Autodesk Inventor part; units mm, degrees
ref_plane "Work Plane1" through (0, 0, 23.8252) normal (0, 0, 1) x (1, 0, 0)
sketch "Sketch1" plane through (0, 0, 0) normal (0, 1, 0) x (-1, 0, 0)
  circle A0 centre (0, 0) radius 30.48
  dimension "d0" = 60.96
extrude "Extrusion1" add sketch "Sketch1" along normal blind 25.4
sketch "Sketch2" plane through (0, 25.4, 0) normal (0, 1, 0) x (1, 0, 0)
  circle A0 centre (0, 0) radius 30.48
  circle A1 centre (0, 0) radius 15.24
  dimension "d3" = 30.48
extrude "Extrusion2" cut sketch "Sketch2" against normal blind 20.828
hole "Hole1" at (0, 25.4, 0) direction (0, -1, 0) diameter 22.225 end through all
ref_plane "Work Plane1" through (0, 0, 23.8252) normal (0, 0, 1) x (1, 0, 0)
hole "Hole2" at (0, 0, 23.8252) direction (0, 1, 0) diameter 5.08 end through all
pattern_circular "Circular Pattern1" count 6 over 360 about axis through (0, 25.4, 0) along (0, -1, 0) of "Hole2"
properties part number ".875 Bearing Hub"
Could you check a few things on this model? Use its own coordinates, in mm. Coordinates: 2 decimals unless noted, no trailing zeros. Write each loop counter-clockwise with the first axis right and the second up, starting at its lowest first coordinate (ties: lowest second). Pieces come first, ordered by that corner, then holes. Notation, with made-up numbers: (-29.75, 25) - (-0.75, 25) arc R24 ccw to (-0.75, 41) - close; hole circle Ø11 at (-0.75, -37). An arc over 180 degrees is marked (long way). Put each result on its own line as item: value. Start each with the question number.
Q1. I want a section at B-B on z = 0. Write out the boundary of the cut face in (x, y).
Q2. I'm going to push flat-ended pins straight in: P1, Ø1, axis at x = 0.5, y = 17.5, coming from the +Z side; P2, Ø6.5, axis at x = 20.63, z = -11.91, coming from the +Y side. Where does each tip first touch, or does it pass through?
Q3. I want a section at C-C on y = 15.5. Write out the boundary of the cut face in (x, z) (1 decimal), plus the area to 3 significant figures.
Q4. Please list where these lines run through material, in increasing order: L1, parallel to Z at x = 0, y = 12.5; L2, parallel to Y at x = 28, z = -11; L3, parallel to X at y = 11, z = 6.
Q5. I want a section at D-D on x = -7. Write out the boundary of the cut face in (y, z).
Q6. I want a section at A-A on x = 0. Write out the boundary of the cut face in (y, z).
Q7. Thinking about a two-plate mould opening in Z: for faces 1 (the cylindrical face through (-3.3, 15.13, 14.88)), 2 (the flat face through (-7, 4.572, -14)), 3 (the cylindrical face through (23.15, 2.32, 11.58)), which applies, pulls with the +Z half, pulls with the -Z half, needs draft (parallel to the pull), parting line crosses it, or undercut?
Checks:
1. outline: (-30.48, 0) - (-11.11, 0) - (-11.11, 25.4) - (-15.24, 25.4) - (-15.24, 4.57) - (-30.48, 4.57) - close; (11.11, 0) - (30.48, 0) - (30.48, 4.57) - (15.24, 4.57) - (15.24, 25.4) - (11.11, 25.4) - close
2. P1: z = 15.24
2. P2: y = 4.57
3. outline: circle Ø30.5 at (0, 0); hole circle Ø22.2 at (0, 0)
3. area: 342 mm²
4. L1: -15.24 to -11.11, 11.11 to 15.24
4. L2: 0 to 4.57
4. L3: -14.01 to -9.35, 9.35 to 14.01
5. outline: (0, -29.67) - (4.57, -29.67) - (4.57, -13.54) - (25.4, -13.54) - (25.4, -8.63) - (0, -8.63) - close; (0, 8.63) - (25.4, 8.63) - (25.4, 13.54) - (4.57, 13.54) - (4.57, 29.67) - (0, 29.67) - close
6. outline: (0, -30.48) - (4.57, -30.48) - (4.57, -26.37) - (0, -26.37) - close; (0, -21.29) - (4.57, -21.29) - (4.57, -15.24) - (25.4, -15.24) - (25.4, -11.11) - (0, -11.11) - close; (0, 11.11) - (25.4, 11.11) - (25.4, 15.24) - (4.57, 15.24) - (4.57, 21.29) - (0, 21.29) - close; (0, 26.37) - (4.57, 26.37) - (4.57, 30.48) - (0, 30.48) - close
7. face 1: parting line crosses it
7. face 2: needs draft
7. face 3: undercut
